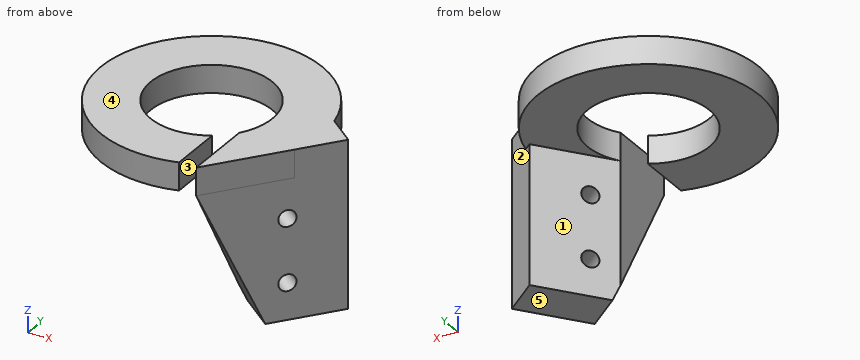
```python
from build123d import *

# Parameters (mm, degrees)
F1_DEPTH      = 6.35
F2_W          = 25.4
F2_H          = 7.62
F3_DEPTH      = 50.8
F3_DEPTH_BACK = 6.35
F4_R          = 1.905
F5_DEPTH      = 25.4
F6_W          = 25.4
F6_H          = 12.7
F7_DEPTH      = 25.4
F9_DEPTH      = 50.8
F11_DEPTH     = 38.1
F12_R         = 1.905
F13_DEPTH     = 25.4
F15_DEPTH     = 25.4


with BuildPart() as f1:
    # F0 (on Top) → F1 (new body)
    with BuildSketch(Plane.XY):
        with BuildLine():
            Line((0, 50.8), (0, 0))
            Line((0, 0), (12.7, 0))
            Line((12.7, 0), (12.7, 50.8))
            ThreePointArc((12.7, 50.8), (-29.065215599, 77.1403437723), (-3.9445899309, 34.6303318914))
            Line((-3.9445899309, 34.6303318914), (-3.9445899309, 47.0864193681))
            ThreePointArc((-3.9445899309, 47.0864193681), (-20.9424468727, 69.0934306211), (0, 50.8))
        make_face()
    extrude(amount=F1_DEPTH)

    # F2 (on face) → F3 (join, two sides)
    with BuildSketch(Plane(origin=(0, 0, 0), x_dir=(1, 0, 0), z_dir=(0, 0, -1))) as f3_sk:
        with Locations((6.35, -3.81)):
            Rectangle(F2_W, F2_H)
    extrude(amount=F3_DEPTH)
    extrude(f3_sk.sketch, amount=-F3_DEPTH_BACK)

    # F4 (on face) → F5 (cut)
    with BuildSketch(Plane.XZ):
        with Locations((6.35, -8.89)):
            Circle(F4_R)
        with Locations((6.35, -23.368)):
            Circle(F4_R)
    extrude(amount=-F5_DEPTH, mode=Mode.SUBTRACT)

    # F6 (on face) → F7 (cut)
    with BuildSketch(Plane(origin=(0, 7.62, 0), x_dir=(-1, 0, 0), z_dir=(0, 1, 0))):
        with Locations((-6.35, -44.45)):
            Rectangle(F6_W, F6_H)
    extrude(amount=-F7_DEPTH, mode=Mode.SUBTRACT)

    # F8 (on face) → F9 (cut)
    with BuildSketch(Plane.XY.offset(6.35)):
        Polygon((12.7, 50.8), (0, 34.6303318914), (0, 17.3151659457), (-24.9700341374, 14.0488371253), (-24.9700341374, -25.5910921842), (41.8248102069, -22.4698372185), (37.4550558627, 0), (37.4550558627, 34.6303318914), align=None)
    extrude(amount=-F9_DEPTH, mode=Mode.SUBTRACT)

    # F10 (on face) → F11 (join)
    with BuildSketch(Plane.XY.offset(6.35)):
        Polygon((0, 50.8), (0, 34.6303318914), (19.6113090693, 59.5994940036), (11.7567067815, 65.7686650951), align=None)
    extrude(amount=-F11_DEPTH)

    # F12 (on face) → F13 (cut)
    with BuildSketch(Plane(origin=(-16.8220820781, 13.2124197576, 0), x_dir=(0.6176790258, 0.7864303027, 0), z_dir=(0.7864303027, -0.6176790258, 0))):
        with Locations((46.2843423936, -8.89)):
            Circle(F12_R)
        with Locations((46.2843423936, -23.368)):
            Circle(F12_R)
    extrude(amount=-F13_DEPTH, mode=Mode.SUBTRACT)

    # F14 (on face) → F15 (cut)
    with BuildSketch(Plane(origin=(-16.8220820781, 13.2124197576, 0), x_dir=(0.6176790258, 0.7864303027, 0), z_dir=(0.7864303027, -0.6176790258, 0))):
        Polygon((27.2343423936, -31.75), (41.6614189744, -31.75), (27.2343423936, 0), align=None)
    extrude(amount=-F15_DEPTH, mode=Mode.SUBTRACT)


solid = f1.part
```
Work out the finished part from the listing and answer in its coordinate system (mm). Face numbers are marked on the shaded views. A direction names the side the tool comes from. Round coordinates to 2 decimals unless told otherwise and drop trailing zeros. Loops run counter-clockwise (first coordinate to the right, second up) from the corner with the lowest first, then second, coordinate; pieces in that order, holes last. Notation, with made-up numbers: (-38.5, 12) -> (-3.5, 12) arc R33 ccw to (-3.5, 47) -> close; hole circle Ø11 at (85.5, -28). An arc over 180 degrees is marked (long way). Write each question's results on one line, items separated by ' | '. Start each with the question number.
1. Given pin 1 Ø3 at (y, z) = (62.5, 1.5) entering from +X; pin 2 Ø5 at (y, z) = (40.5, -18.5) entering from -X; pin 3 Ø2 at (y, z) = (65.5, -10) entering from +X, each flat-ended and moving along its own axis, determine where each tip first touches the part or whether it passes through.
2. Find the intervals of material crossed by probe 1 along Y at (x, z) = (-12, 1.5); probe 2 along Z at (x, y) = (9, 54); probe 3 along Z at (x, y) = (-22, 49), in increasing order. Write a range as from..to.
3. Section A-A (y = 58.5) is taken. Determine the outline of the cut face in (x, z), plus the area to 3 significant figures.
4. A tool of negligible diameter and unlimited length cuts with its end or side. For the marked faces 1, 2, 3, 4 and 5, from which of +Z, -Z, +X, -X, +Y, -Y can it reach the whole face along a straight path? Write none if from no direction.
5. Section C-C (x = -19.5) is taken. Determine the outline of the cut face in (y, z), plus the area to 3 significant figures.
6. Section B-B (z = -10) is taken. Determine the outline of the cut face in (x, y), plus the area to 3 significant figures.
7. Section D-D (z = -17) is taken. Determine the outline of the cut face in (x, y), plus the area to 3 significant figures.
Evaluation:
1) pin 1: stops at x = 17.83 | pin 2: stops at x = 2.46 | pin 3: stops at x = 13.37
2) probe 1: y = 33.53..44.97, 72.88..84.31 | probe 2: z = -31.75..-24.14, -22.6..-9.66, -8.12..6.35 | probe 3: z = 0..6.35
3) outline: (-36.76, 0) -> (-25.33, 0) -> (-25.33, 6.35) -> (-36.76, 6.35) -> close; (2.6, 0) -> (6.05, 0) -> (6.05, -31.75) -> (18.75, -31.75) -> (18.75, 6.35) -> (2.6, 6.35) -> close | area: 578 mm2
4) face 1: -Z, -X, +Y | face 2: -Z, +X, +Y | face 3: +Z, -Z, -Y | face 4: +Z, +X, -X, +Y, -Y | face 5: -Z, +X, -X, +Y, -Y
5) outline: (34.86, 0) -> (47.56, 0) -> (47.56, 6.35) -> (34.86, 6.35) -> close; (70.28, 0) -> (82.98, 0) -> (82.98, 6.35) -> (70.28, 6.35) -> close | area: 161 mm2
6) outline: (0, 40.41) -> (2.81, 38.2) -> (10.81, 48.39) -> (2.96, 54.56) -> (0, 50.8) -> close; (4.87, 57) -> (12.72, 50.83) -> (19.61, 59.6) -> (11.76, 65.77) -> close | area: 215 mm2
7) outline: (0, 44.45) -> (4.77, 40.71) -> (19.61, 59.6) -> (11.76, 65.77) -> (0, 50.8) -> close | area: 230 mm2
